from build123d import *

# Parameters (mm, degrees)
F3_DEPTH = 75.32841


with BuildPart() as f1:
    # F0 (on Top) → F1 (revolve)
    with BuildSketch(Plane.XY):
        Polygon((75.32841, 25.4), (75.32841, 34.29), (55.00841, 34.29), (55.00841, 40.64), (64.604973, 50.236563), (57.420768, 57.420768), (30.48, 30.48), (30.48, 25.4), align=None)
    revolve(axis=Axis((1.895559, 0, 0), (1, 0, 0)))

    # F2 (on Right) → F3 (cut, through all)
    with BuildSketch(Plane.YZ):
        with BuildLine():
            ThreePointArc((-3.81, 25.112624), (0, 25.4), (3.81, 25.112624))
            Line((3.81, 25.112624), (3.81, 27.94))
            Line((3.81, 27.94), (-3.81, 27.94))
            Line((-3.81, 27.94), (-3.81, 25.112624))
        make_face()
    extrude(amount=F3_DEPTH, mode=Mode.SUBTRACT)


solid = f1.part
Check sheet for the modelled part. Datum: model origin and axes. Units: mm. A direction names the side the tool comes from. Give positions to 0.01 mm unless a question says otherwise; leave off trailing zeros. Loops run counter-clockwise (first coordinate to the right, second up) from the corner with the lowest first, then second, coordinate; pieces in that order, holes last. Notation, with made-up numbers: M -9,7.25 L 18,7.25 A15 cw 18,35.25 Z; hole C 36.25,28 d5. An arc over 180 degrees is marked long. Answer as a JSON object with one key per item and string values. Group by question number.
Q1. Release check for a two-part mould opening along Y. For faces 1 (the flat face through (75.328, 26, -2)), 2 (the flat face through (55.008, 18, -30)), 3 (the conical face through (31.788, 29.364, -12.175)) record: released by +Y, released by -Y, zero draft, split by the parting line, or undercut.
Q2. Material ranges on line 1 along Z through (x, y) = (57.5, 38); line 2 along Z through (x, y) = (60.5, -14.5); line 3 along Z through (x, y) = (56, 0), recorded low to high. Write a range as [from, to].
Q3. Go/stop test with flat-tipped pins: P1, Ø1, axis at x = 49, y = -25.5, coming from the +Z side; P2, Ø6, axis at x = 39, z = -2, coming from the -Y side; P3, Ø2.5, axis at x = 63, y = 0, coming from the -Z side. Record where each tip stops, or that it passes through.
Q4. Cross-section at B-B on z = 0. Record the cut outline in (x, y), then the cut area to 3 significant figures.
Q5. Cross-section at A-A on y = 0. Record the cut outline in (x, z).
Q6. Cross-section at C-C on x = 51. Record the cut outline in (y, z), then the cut area to 3 significant figures.
Q7. Access from +Z, -Z, +X, -X, +Y, -Y to the whole of each face (thin tool, end or side, straight path). Record for faces 4 (the cylindrical face through (65.026, 18.434, 28.913)), 5 (the flat face through (30.48, -7, -25)), 6 (the flat face through (53, 0, 27.94)).
Evaluation:
{
 "1": {"face 1": "zero draft", "face 2": "undercut", "face 3": "split by the parting line"},
 "2": {"line 1": "z = [-42.94, -20.4], [20.4, 42.94]", "line 2": "z = [-52.37, -43.79], [-31.07, -20.85], [20.85, 31.07], [43.79, 52.37]", "line 3": "z = [-56, -41.63], [-34.29, -25.4], [27.94, 34.29], [41.63, 56]"},
 "3": {"P1": "stops at z = 42.5", "P2": "stops at y = -41.96", "P3": "stops at z = -53.09"},
 "4": {"outline": "M 30.48,-30.48 L 57.42,-57.42 L 64.6,-50.24 L 55.01,-40.64 L 55.01,-34.29 L 75.33,-34.29 L 75.33,-25.4 L 30.48,-25.4 Z; M 30.48,25.4 L 75.33,25.4 L 75.33,34.29 L 55.01,34.29 L 55.01,40.64 L 64.6,50.24 L 57.42,57.42 L 30.48,30.48 Z", "area": "1,380 mm2"},
 "5": {"outline": "M 30.48,-30.48 L 57.42,-57.42 L 64.6,-50.24 L 55.01,-40.64 L 55.01,-34.29 L 75.33,-34.29 L 75.33,-25.4 L 30.48,-25.4 Z; M 30.48,27.94 L 75.33,27.94 L 75.33,34.29 L 55.01,34.29 L 55.01,40.64 L 64.6,50.24 L 57.42,57.42 L 30.48,30.48 Z"},
 "6": {"outline": "C 0,0 d102; hole M -3.81,25.11 A25.4 ccw long 3.81,25.11 L 3.81,27.94 L -3.81,27.94 Z", "area": "6,120 mm2"},
 "7": {"face 4": "+X", "face 5": "+Z, -Z, -X, +Y, -Y", "face 6": "+X, -X"}
}
